```python
from build123d import *

# Parameters (mm, degrees)
SKETCH6_W               = 5
SKETCH6_H               = 30
SKETCH7_R               = 15
BOSS_EXTRUDE1_DEPTH     = 10
CUT_EXTRUDE1_DEPTH      = 281.256736501
CUT_EXTRUDE1_DEPTH_BACK = 281.256736501
SKETCH7_3_W             = 15
SKETCH7_3_H             = 15
FILLET1_R               = 10
FILLET2_R               = 15
SKETCH9_R               = 10.5
BOSS_EXTRUDE2_DEPTH     = 120


with BuildPart() as part:
    # Sweep1: sweep along a path in Sketch2
    with BuildLine(Plane(origin=(0, 0, 0), x_dir=(1, 0, 0), z_dir=(0, 1, 0))) as sweep1_path:
        Line((0, -75), (0, 75))
        Line((0, 75), (49.497474683, 124.497474683))
        Line((49.497474683, 124.497474683), (49.497474683, 274.497474683))
    # Sketch6 → Sweep1 (sweep)
    with BuildSketch(Plane.XY.offset(75)):
        Rectangle(SKETCH6_W, SKETCH6_H)
    sweep(path=sweep1_path.line, transition=Transition.RIGHT)

    # Sketch7 → Boss-Extrude1 (add)
    with BuildSketch(Plane.ZY.offset(2.5)):
        with Locations(Location((60, 0, 0), (0, 0, 270))):
            Circle(SKETCH7_R)
    extrude(amount=BOSS_EXTRUDE1_DEPTH)

    # Sketch7<3> → Cut-Extrude1 (cut, two sides: drawn at the far end of the back side and taken through both)
    with BuildSketch(Plane.ZY.offset(2.5).offset(-CUT_EXTRUDE1_DEPTH_BACK)):
        with Locations((60, 0)):
            Rectangle(SKETCH7_3_W, SKETCH7_3_H)
    extrude(amount=CUT_EXTRUDE1_DEPTH + CUT_EXTRUDE1_DEPTH_BACK, mode=Mode.SUBTRACT)

    # Fillet1
    fillet1_edges = [part.edges().sort_by_distance(p)[0] for p in [
        (-2.5, 0, -76.035533906),
        (2.5, 0, -73.964466094),
        (51.997474683, 0, -123.461940777),
        (46.997474683, 0, -125.533008589),
    ]]
    fillet(fillet1_edges, radius=FILLET1_R)

    # Fillet2
    fillet2_edges = [part.edges().sort_by_distance(p)[0] for p in [
        (0, 15, 75),
        (0, -15, 75),
        (49.497474683, -15, -274.497474683),
        (49.497474683, 15, -274.497474683),
    ]]
    fillet(fillet2_edges, radius=FILLET2_R - 0.0001)  # a hair under: the kernel refuses the full size

    # Sketch9 → Boss-Extrude2 (add)
    with BuildSketch(Plane(origin=(51.997474683, 0, 0), x_dir=(0, 0, -1), z_dir=(1, 0, 0))):
        with Locations(Location((259.497474683, 0, 0), (0, 0, 90))):
            Circle(SKETCH9_R)
    extrude(amount=BOSS_EXTRUDE2_DEPTH)


solid = part.part
```
Here's how the part is built. I have some questions about the finished solid (model axes, mm). A direction names the side the tool comes from. Coordinates: 2 decimals unless noted, no trailing zeros. Order: outer loops, then holes, each group sorted by start corner. A loop starts at its lowest first (then second) coordinate and runs counter-clockwise, first axis right, second up. Notation, with made-up numbers: (-16.75, 40.5) -> (13.25, 40.5) arc R3 ccw to (13.25, 45.5) -> close; hole circle Ø5 at (26, 42). An arc over 180 degrees is marked (long way). Return JSON: item names as keys, results as strings.
1) I'm going to push flat-ended pins straight in: P1, Ø3, axis at x = 100, y = -6.5, coming from the +Z side; P2, Ø5, axis at x = 113.5, y = -6, coming from the -Z side; P3, Ø1.5, axis at x = 85, y = -2.5, coming from the +Z side. Where does each tip first touch, or does it pass through?
Conclusion:
{"P1": "stops at z = -250.26", "P2": "stops at z = -269.4", "P3": "stops at z = -249.14"}
2) If we section it at B-B on x = 26.5: List the corners of the cut face in (y, z) for me.
Conclusion:
{"outline": "(-15, -105.04) -> (15, -105.04) -> (15, -97.96) -> (-15, -97.96) -> close"}
3) If I drill on probe 1 along X at (y, z) = (-13, 30); probe 2 along X at (y, z) = (6, -148.5); probe 3 along Z at (x, y) = (128.5, 8), over which ranges is the centre line in solid material (lowest first)?
Conclusion:
{"probe 1": "x = -2.5 to 2.5", "probe 2": "x = 47 to 52", "probe 3": "z = -266.3 to -252.7"}
4) If we section it at A-A on z = -148: List the corners of the cut face in (x, y) for me, plus the area to 3 significant figures.
Conclusion:
{"outline": "(47, -15) -> (52, -15) -> (52, 15) -> (47, 15) -> close", "area": "150 mm²"}
5) Thinking about a two-plate mould opening in Z: for faces 4 (the flat face through (35, 15, -112)), 5 (the flat face through (-5, -7.5, 60)), 6 (the cylindrical face through (111.157, -1.367, -249.087)), which applies, +Z half, -Z half, draft (parallel to the pull), parting line (faces both ways), or undercut?
Conclusion:
{"face 4": "draft", "face 5": "undercut", "face 6": "parting line"}
6) On a 3-axis mill with a long thin cutter (end or side, diameter ignored), from which of +Z, -Z, +X, -X, +Y, -Y can I reach the whole of each face in a straight line? I mean faces 1 (the flat face through (2.5, 0, 2)), 2 (the cylindrical face through (-7.43, 3.252, 45.357)), 3 (the flat face through (-5, 7.5, 60)). Say none if no direction works.
Conclusion:
{"face 1": "+Z, +X, +Y, -Y", "face 2": "-X", "face 3": "+X, -X"}
